```python
from build123d import *

# Parameters (mm, degrees)
SKETCH1_R           = 6.5
SKETCH1_R_2         = 2
BOSS_EXTRUDE1_DEPTH = 4
CHAMFER1_SIZE       = 0.5


with BuildPart() as part:
    # Sketch1 → Boss-Extrude1 (new body)
    with BuildSketch(Plane(origin=(0, 0, 0), x_dir=(1, 0, 0), z_dir=(0, 1, 0))):
        Circle(SKETCH1_R)
        Circle(SKETCH1_R_2, mode=Mode.SUBTRACT)
    extrude(amount=BOSS_EXTRUDE1_DEPTH)

    # Sketch2 → Cut-Revolve1 (revolve, cut)
    with BuildSketch(Plane(origin=(0, 0, 0), x_dir=(0, 0, -1), z_dir=(1, 0, 0))):
        Polygon((-6.5, 3), (-6.5, 1), (-5.5, 2), align=None)
    revolve(axis=Axis((0, 4, 0), (0, -1, 0)), mode=Mode.SUBTRACT)

    # Chamfer1
    chamfer1_edges = [part.edges().sort_by_distance(p)[0] for p in [
        (-6.5, 0, 0),
        (-6.5, 4, 0),
        (-2, 0, 0),
        (-2, 4, 0),
    ]]
    chamfer(chamfer1_edges, length=CHAMFER1_SIZE)


solid = part.part
```
The listing builds one solid part. Answer for the finished solid, in the listing's coordinates (mm). Give positions to 0.01 mm unless a question says otherwise; leave off trailing zeros. Order: outer loops, then holes, each group sorted by start corner. A loop starts at its lowest first (then second) coordinate and runs counter-clockwise, first axis right, second up. Notation, with made-up numbers: (-8, -38) -> (42, -38) arc R21 ccw to (42, -5) -> close; hole circle Ø1 at (72, 65.25). An arc over 180 degrees is marked (long way). One line per item, written item: value.
1) Find section C-C, the plane y = 1.3. Determine the outline of the cut face in (x, z), plus the area to 3 significant figures.
Reported:
outline: circle Ø12.4 at (0, 0); hole circle Ø4 at (0, 0)
area: 108 mm^2
2) Find section B-B, the plane z = 0. Determine the outline of the cut face in (x, y), plus the area to 3 significant figures.
Reported:
outline: (-6.5, 0.5) -> (-6, 0) -> (-2.5, 0) -> (-2, 0.5) -> (-2, 3.5) -> (-2.5, 4) -> (-6, 4) -> (-6.5, 3.5) -> (-6.5, 3) -> (-5.5, 2) -> (-6.5, 1) -> close; (2, 0.5) -> (2.5, 0) -> (6, 0) -> (6.5, 0.5) -> (6.5, 1) -> (5.5, 2) -> (6.5, 3) -> (6.5, 3.5) -> (6, 4) -> (2.5, 4) -> (2, 3.5) -> close
area: 33.0 mm^2
3) Flat-ended cylindrical pins translate along their axes: P1, Ø2, axis at x = -4.5, y = 3.5, coming from the -Z side; P2, Ø2.5, axis at x = 0, z = 0, coming from the +Y side. Find the tip coordinate at first contact, or state that the pin passes through.
Reported:
P1: stops at z = -5.48
P2: passes through
4) Find the intervals of material crossed by line 1 (Z direction, x = 0.75, y = 2.7); line 2 (X direction, y = 3.55, z = -1.25); line 3 (X direction, y = 2.3, z = 0), in increasing order.
Reported:
line 1: z = -6.15 to -1.85, 1.85 to 6.15
line 2: x = -6.33 to -1.62, 1.62 to 6.33
line 3: x = -5.8 to -2, 2 to 5.8
5) Find section A-A, the plane x = 0. Determine the outline of the cut face in (y, z), plus the area to 3 significant figures.
Reported:
outline: (0, -6) -> (0.5, -6.5) -> (1, -6.5) -> (2, -5.5) -> (3, -6.5) -> (3.5, -6.5) -> (4, -6) -> (4, -2.5) -> (3.5, -2) -> (0.5, -2) -> (0, -2.5) -> close; (0, 2.5) -> (0.5, 2) -> (3.5, 2) -> (4, 2.5) -> (4, 6) -> (3.5, 6.5) -> (3, 6.5) -> (2, 5.5) -> (1, 6.5) -> (0.5, 6.5) -> (0, 6) -> close
area: 33.0 mm^2
